Can you work these out from the model? Positions are in its coordinate system, mm. A direction names the side the tool comes from. Round coordinates to 2 decimals unless told otherwise and drop trailing zeros. Loops run counter-clockwise (first coordinate to the right, second up) from the corner with the lowest first, then second, coordinate; pieces in that order, holes last. Notation, with made-up numbers: (44.5, -38) - (49.5, -38) arc R4 ccw to (49.5, -31) - close; hole circle Ø1 at (26.5, 83.25). An arc over 180 degrees is marked (long way). Answer as CSV lines item,"result".
```python
from build123d import *

# Parameters (mm, degrees)
BOSS_EXTRUDE4_DEPTH = 2.5
SKETCH7_R           = 11
CUT_EXTRUDE1_DEPTH  = 6
SKETCH8_R           = 14
SKETCH8_R_2         = 12
BOSS_EXTRUDE5_DEPTH = 2
FILLET1_R           = 2


with BuildPart() as part:
    # Sketch6 → Boss-Extrude4 (new body, symmetric)
    with BuildSketch(Plane.XY):
        with BuildLine():
            Line((-32.469344609, 53), (-16.469344609, 65))
            ThreePointArc((-16.469344609, 65), (0, 70.489781536), (16.469344609, 65))
            Line((16.469344609, 65), (32.469344609, 53))
            ThreePointArc((32.469344609, 53), (35.413616519, 49.472135955), (36.469344609, 45))
            Line((36.469344609, 45), (36.469344609, -44.226497308))
            ThreePointArc((36.469344609, -44.226497308), (35.129598647, -49.226497308), (31.469344609, -52.886751346))
            Line((31.469344609, -52.886751346), (19.148836533, -60))
            ThreePointArc((19.148836533, -60), (0, -65.130915285), (-19.148836533, -60))
            Line((-19.148836533, -60), (-31.469344609, -52.886751346))
            ThreePointArc((-31.469344609, -52.886751346), (-35.129598647, -49.226497308), (-36.469344609, -44.226497308))
            Line((-36.469344609, -44.226497308), (-36.469344609, 45))
            ThreePointArc((-36.469344609, 45), (-35.413616519, 49.472135955), (-32.469344609, 53))
        make_face()
    extrude(amount=BOSS_EXTRUDE4_DEPTH, both=True)

    # Sketch7 → Cut-Extrude1 (cut, through all)
    with BuildSketch(Plane.XY.offset(2.5)):
        with Locations((15, -19.159106742)):
            Circle(SKETCH7_R)
        with Locations((-15, -19.159106742)):
            Circle(SKETCH7_R)
        with Locations((-15, 20)):
            Circle(SKETCH7_R)
        with Locations((15, 20)):
            Circle(SKETCH7_R)
    extrude(amount=-CUT_EXTRUDE1_DEPTH, mode=Mode.SUBTRACT)

    # Sketch8 → Boss-Extrude5 (add)
    with BuildSketch(Plane.XY.offset(2.5)):
        with Locations((15, -19.159106742)):
            Circle(SKETCH8_R)
        with Locations((15, -19.159106742)):
            Circle(SKETCH8_R_2, mode=Mode.SUBTRACT)
        with Locations((-15, 20)):
            Circle(SKETCH8_R)
        with Locations((-15, 20)):
            Circle(SKETCH8_R_2, mode=Mode.SUBTRACT)
        with Locations((15, 20)):
            Circle(SKETCH8_R)
        with Locations((15, 20)):
            Circle(SKETCH8_R_2, mode=Mode.SUBTRACT)
        with Locations((-15, -19.159106742)):
            Circle(SKETCH8_R)
        with Locations((-15, -19.159106742)):
            Circle(SKETCH8_R_2, mode=Mode.SUBTRACT)
    extrude(amount=BOSS_EXTRUDE5_DEPTH)

    # Fillet1
    fillet1_edges = [part.edges().sort_by_distance(p)[0] for p in [
        (-35.413616519, 49.472135955, 2.5),
        (-36.469344609, 0.386751346, 2.5),
        (-35.129598647, -49.226497308, 2.5),
        (-25.309090571, -56.443375673, 2.5),
        (0, -65.130915285, 2.5),
        (25.309090571, -56.443375673, 2.5),
        (35.129598647, -49.226497308, 2.5),
        (36.469344609, 0.386751346, 2.5),
        (35.413616519, 49.472135955, 2.5),
        (24.469344609, 59, 2.5),
        (0, 70.489781536, 2.5),
        (-24.469344609, 59, 2.5),
    ]]
    fillet(fillet1_edges, radius=FILLET1_R)


solid = part.part
```
Q1. On a 3-axis mill with a long thin cutter (end or side, diameter ignored), from which of +Z, -Z, +X, -X, +Y, -Y can I reach the whole of each face in a straight line? I mean faces 1 (the cylindrical face through (0.28, -65.13, -0.98)), 2 (the flat face through (5, 15, 2.5)). Say none if no direction works.
Checks:
face 1,"+Z, -Z, -Y"
face 2,"+Z"
Q2. I'm going to push flat-ended pins straight in: pin 1 Ø12 at (x, y) = (9.5, 20.5) entering from +Z; pin 2 Ø1 at (x, z) = (-19, -0.5) entering from -Y; pin 3 Ø1.5 at (y, z) = (-50, 0.5) entering from -X. Where does each tip first touch, or does it pass through?
Checks:
pin 1,"z = 2.5"
pin 2,"y = -60.37"
pin 3,"x = -35.12"
Q3. If I drill on line 1 along Y through (x, z) = (15, 0.7); line 2 along Y through (x, z) = (15, 3.95); line 3 along X through (y, z) = (19, 1.75), over which ranges is the centre line in solid material (lowest first)? Write a range as [from, to].
Checks:
line 1,"[-62.06, -30.16], [-8.16, 9], [31, 66.02]"
line 2,"[-33.16, -31.16], [-7.16, -5.16], [6, 8], [32, 34]"
line 3,"[-36.03, -25.95], [-4.05, 4.05], [25.95, 36.03]"
Q4. We'd pull the mould along Y, two halves only. Please class faces 3 (the flat face through (25.4, -56.39, -0.98)), 4 (the cylindrical face through (27.932, -24.521, 3.486)), 5 (the flat face through (-11, -31, 4.5)), 6 (the flat face through (4, -23, 2.5)): pulls with the +Y half, pulls with the -Y half, needs draft (parallel to the pull), parting line crosses it, or undercut.
Checks:
face 3,"pulls with the -Y half"
face 4,"undercut"
face 5,"needs draft"
face 6,"undercut"
Q5. Imagine slicing it at C-C (y = -2). Write out the boundary of the cut face in (x, z), then the cut area to 3 significant figures.
Checks:
outline,"(-36.47, -2.5) - (36.47, -2.5) - (36.47, 0.5) arc R2 ccw to (34.47, 2.5) - (-34.47, 2.5) arc R2 ccw to (-36.47, 0.5) - close"
area,"363 mm²"
Q6. Imagine slicing it at A-A (y = 20). Count the separate pieces of the cut face and the enclosed holes in it, then the cut area to 3 significant figures.
Checks:
separate pieces,"3"
enclosed holes,"0"
area,"159 mm²"
